```python
from build123d import *

# Parameters (mm, degrees)
F0_W     = 75
F0_H     = 25
F1_DEPTH = 3
F2_R     = 2.5
F3_DEPTH = 5
F4_R     = 1
F5_DEPTH = 3


with BuildPart() as f1:
    # F0 (on Top) → F1 (new body)
    with BuildSketch(Plane.XY):
        with Locations((0.05, -0.046321)):
            Rectangle(F0_W, F0_H)
    extrude(amount=F1_DEPTH)

    # F2 (on Top) → F3 (join)
    with BuildSketch(Plane.XY):
        with Locations((-24.999432, 0)):
            Circle(F2_R)
        with Locations((-8.305821, 0)):
            Circle(F2_R)
        with Locations((8.388246, 0)):
            Circle(F2_R)
        with Locations((25.083415, 0)):
            Circle(F2_R)
    extrude(amount=F3_DEPTH)

    # F4 (on face) → F5 (cut)
    with BuildSketch(Plane.XY.offset(5)):
        with Locations((-24.999432, 0)):
            Circle(F4_R)
        with Locations((-8.304862, 0)):
            Circle(F4_R)
        with Locations((8.406557, 0)):
            Circle(F4_R)
        with Locations((25.101803, 0)):
            Circle(F4_R)
    extrude(amount=-F5_DEPTH, mode=Mode.SUBTRACT)


solid = f1.part
```
Here's how the part is built. I have some questions about the finished solid (model axes, mm). A direction names the side the tool comes from. Round coordinates to 2 decimals unless told otherwise and drop trailing zeros. Order: outer loops, then holes, each group sorted by start corner. A loop starts at its lowest first (then second) coordinate and runs counter-clockwise, first axis right, second up. Notation, with made-up numbers: (50.5, 8.5) -> (57.5, 8.5) arc R26 ccw to (57.5, 31.5) -> close; hole circle Ø7 at (81.25, 48.5). An arc over 180 degrees is marked (long way). Use a Markdown table: item, result. Add a question column.
(1) Suppose I cut it at C-C, the plane y = 5. Please give me the cut outline in (x, z), and give its area (3 significant figures).
(2) Suppose I cut it at B-B, the plane x = 33. Please give me the cut outline in (y, z), and give its area (3 significant figures).
(3) I need wall thicknesses on line 1 along Z through (x, y) = (10.5, 9). Which ranges of the line are inside material? Lowest first, please.
(4) Suppose I cut it at A-A, the plane z = 3.75. Please give me the cut outline in (x, y).
(5) If we mould it in two halves opening along X, with no side actions, what happens to faces 3 (the face through (0, 0, 0)), 4 (the face through (-10.803, 0.11, 3.986)), 5 (the face through (-37.45, 0, 1)), 6 (the face through (37.55, 0, 1))? For each: released by +X, released by -X, zero draft, split by the parting line, or undercut.
(6) For faces 1 (the face through (-27.497, 0.11, 3.986)), 2 (the face through (26, -1, 5)), which set-ups out of +Z, -Z, +X, -X, +Y, -Y let a thin tool reach every point of the face, with its end or its side?
(7) For pin 1 Ø0.6 at (x, y) = (25, 0) entering from +Z; pin 2 Ø2.5 at (x, y) = (-8.3, 0) entering from -Z; pin 3 Ø1.5 at (y, z) = (4, 4.5) entering from -X; pin 4 Ø5 at (x, y) = (17, -2.5) entering from +Z, each with a flat end and sliding along its axis, tell me the tip position at first contact or that it passes through.
Verdict:
| question | item | result |
|---|---|---|
| 1 | outline | (-37.45, 0) -> (37.55, 0) -> (37.55, 3) -> (-37.45, 3) -> close |
| 1 | area | 225 mm2 |
| 2 | outline | (-12.55, 0) -> (12.45, 0) -> (12.45, 3) -> (-12.55, 3) -> close |
| 2 | area | 75.0 mm2 |
| 3 | line 1 | 0 to 3 |
| 4 | outline | circle Ø5 at (-25, 0); circle Ø5 at (-8.31, 0); circle Ø5 at (8.39, 0); circle Ø5 at (25.08, 0); hole circle Ø2 at (-25, 0); hole circle Ø2 at (-8.3, 0); hole circle Ø2 at (8.41, 0); hole circle Ø2 at (25.1, 0) |
| 5 | face 3 | zero draft |
| 5 | face 4 | undercut |
| 5 | face 5 | released by -X |
| 5 | face 6 | released by +X |
| 6 | face 1 | +Z |
| 6 | face 2 | +Z, +X, -X, +Y, -Y |
| 7 | pin 1 | z = 2 |
| 7 | pin 2 | z = 0 |
| 7 | pin 3 | through |
| 7 | pin 4 | z = 3 |
